```python
from build123d import *

# Parameters (mm, degrees)
BOSS_EXTRUDE2_DEPTH = 2.8956


with BuildPart() as part:
    # Sketch1 → Boss-Extrude2 (new body)
    with BuildSketch(Plane(origin=(0, 0, 0), x_dir=(1, 0, 0), z_dir=(0, 1, 0))):
        with BuildLine():
            Line((21.59, 1.2446), (25.393976036, 1.2446))
            add(Edge.make_bspline(
                [(25.393976036, 1.2446), (25.305125525, 10.422131382), (23.943355437, 19.0754)],
                knots=[4.73416848, 4.73416848, 4.73416848, 5.052697334, 5.052697334, 5.052697334], degree=2, weights=[1, 0.987344206, 1]))
            Line((23.943355437, 19.0754), (19.930240776, 19.0754))
            Line((19.930240776, 19.0754), (19.930240776, 21.5646))
            Line((19.930240776, 21.5646), (23.522368768, 21.5646))
            add(Edge.make_bspline(
                [(23.522368768, 21.5646), (17.413838434, 55.296547713), (1.2446, 57.081350193)],
                knots=[5.099304053, 5.099304053, 5.099304053, 6.234165678, 6.234165678, 6.234165678], degree=2, weights=[1, 0.843284611, 1]))
            Line((1.2446, 57.081350193), (1.2446, 53.34))
            Line((1.2446, 53.34), (-1.2446, 53.34))
            Line((-1.2446, 53.34), (-1.2446, 57.081350193))
            add(Edge.make_bspline(
                [(-1.2446, 57.081350193), (-17.413838434, 55.296547713), (-23.522368768, 21.5646)],
                knots=[0.049019629, 0.049019629, 0.049019629, 1.183881254, 1.183881254, 1.183881254], degree=2, weights=[1, 0.843284611, 1]))
            Line((-23.522368768, 21.5646), (-19.930240776, 21.5646))
            Line((-19.930240776, 21.5646), (-19.930240776, 19.0754))
            Line((-19.930240776, 19.0754), (-23.943355437, 19.0754))
            add(Edge.make_bspline(
                [(-23.943355437, 19.0754), (-25.305125525, 10.422131382), (-25.393976036, 1.2446)],
                knots=[1.230487974, 1.230487974, 1.230487974, 1.549016827, 1.549016827, 1.549016827], degree=2, weights=[1, 0.987344206, 1]))
            Line((-25.393976036, 1.2446), (-21.59, 1.2446))
            Line((-21.59, 1.2446), (-21.59, -1.2446))
            Line((-21.59, -1.2446), (-25.393976036, -1.2446))
            add(Edge.make_bspline(
                [(-25.393976036, -1.2446), (-25.305125525, -10.422131382), (-23.943355437, -19.0754)],
                knots=[1.592575826, 1.592575826, 1.592575826, 1.91110468, 1.91110468, 1.91110468], degree=2, weights=[1, 0.987344206, 1]))
            Line((-23.943355437, -19.0754), (-19.930240776, -19.0754))
            Line((-19.930240776, -19.0754), (-19.930240776, -21.5646))
            Line((-19.930240776, -21.5646), (-23.522368768, -21.5646))
            add(Edge.make_bspline(
                [(-23.522368768, -21.5646), (-22.395811131, -27.785569894), (-20.658836503, -33.249220312)],
                knots=[1.957711399, 1.957711399, 1.957711399, 2.191722412, 2.191722412, 2.191722412], degree=2, weights=[1, 0.993162662, 1]))
            Line((-20.658836503, -33.249220312), (-40.656934115, -75.189915873))
            ThreePointArc((-40.656934115, -75.189915873), (-40.089838211, -78.146952179), (-37.097948163, -78.484969079))
            Line((-37.097948163, -78.484969079), (-8.029094451, -54.219568092))
            add(Edge.make_bspline(
                [(-8.029094451, -54.219568092), (0, -60.238814416), (8.029094451, -54.219568092)],
                knots=[2.819970364, 2.819970364, 2.819970364, 3.463214943, 3.463214943, 3.463214943], degree=2, weights=[1, 0.948723851, 1]))
            Line((8.029094451, -54.219568092), (37.097948163, -78.484969079))
            ThreePointArc((37.097948163, -78.484969079), (40.089838211, -78.146952179), (40.656934115, -75.189915873))
            Line((40.656934115, -75.189915873), (20.658836503, -33.249220312))
            add(Edge.make_bspline(
                [(20.658836503, -33.249220312), (22.395811131, -27.785569894), (23.522368768, -21.5646)],
                knots=[4.091462895, 4.091462895, 4.091462895, 4.325473908, 4.325473908, 4.325473908], degree=2, weights=[1, 0.993162662, 1]))
            Line((23.522368768, -21.5646), (19.930240776, -21.5646))
            Line((19.930240776, -21.5646), (19.930240776, -19.0754))
            Line((19.930240776, -19.0754), (23.943355437, -19.0754))
            add(Edge.make_bspline(
                [(23.943355437, -19.0754), (25.305125525, -10.422131382), (25.393976036, -1.2446)],
                knots=[4.372080627, 4.372080627, 4.372080627, 4.690609481, 4.690609481, 4.690609481], degree=2, weights=[1, 0.987344206, 1]))
            Line((25.393976036, -1.2446), (21.59, -1.2446))
            Line((21.59, -1.2446), (21.59, 1.2446))
        make_face()
        with BuildLine():
            Line((-14.613224312, -41.884600001), (-10.124198394, -41.884600001))
            add(Edge.make_bspline(
                [(0, -50.8), (-0.374242122, -50.8), (-1.087449753, -50.722280744), (-2.740425126, -50.190283538), (-5.318112389, -48.514264833), (-8.117471478, -45.20633596), (-9.696301311, -42.637606864), (-10.124198394, -41.884600001)],
                knots=[-3.141592654, -3.141592654, -3.141592654, -3.141592654, -3.043417883, -2.945243113, -2.748893572, -2.552544031, -2.478028469, -2.478028469, -2.478028469, -2.478028469], degree=3))
            add(Edge.make_bspline(
                [(0, -50.8), (0.374242122, -50.8), (1.087449753, -50.722280744), (2.740425126, -50.190283538), (5.318112389, -48.514264833), (8.117471478, -45.20633596), (9.696301311, -42.637606864), (10.124198394, -41.884600001)],
                knots=[-3.141592654, -3.141592654, -3.141592654, -3.141592654, -3.043417883, -2.945243113, -2.748893572, -2.552544031, -2.478028469, -2.478028469, -2.478028469, -2.478028469], degree=3))
            Line((10.124198394, -41.884600001), (14.613224312, -41.884600001))
            Line((14.613224312, -41.884600001), (14.613224312, -39.395400001))
            Line((14.613224312, -39.395400001), (11.431305901, -39.395400001))
            add(Edge.make_bspline(
                [(11.431305901, -39.395400001), (11.677149239, -38.889598832), (12.987812642, -36.070874709), (15.148196965, -30.166196648), (18.099752632, -17.775460251), (19.683498245, 0), (18.099752632, 17.775460251), (15.148196965, 30.166196648), (12.987812642, 36.070874709), (11.677149239, 38.889598832), (11.431305901, 39.395400001)],
                knots=[-2.400745736, -2.400745736, -2.400745736, -2.400745736, -2.35619449, -2.159844949, -1.963495408, -1.570796327, -1.178097245, -0.981747704, -0.785398163, -0.740846918, -0.740846918, -0.740846918, -0.740846918], degree=3))
            Line((11.431305901, 39.395400001), (14.613224312, 39.395400001))
            Line((14.613224312, 39.395400001), (14.613224312, 41.884600001))
            Line((14.613224312, 41.884600001), (10.124198394, 41.884600001))
            add(Edge.make_bspline(
                [(10.124198394, 41.884600001), (9.696301311, 42.637606864), (8.117471478, 45.20633596), (5.318112389, 48.514264833), (2.740425126, 50.190283538), (1.087449753, 50.722280744), (0.374242122, 50.8), (0, 50.8)],
                knots=[-0.663564185, -0.663564185, -0.663564185, -0.663564185, -0.589048623, -0.392699082, -0.196349541, -0.09817477, 0, 0, 0, 0], degree=3))
            add(Edge.make_bspline(
                [(-10.124198394, 41.884600001), (-9.696301311, 42.637606864), (-8.117471478, 45.20633596), (-5.318112389, 48.514264833), (-2.740425126, 50.190283538), (-1.087449753, 50.722280744), (-0.374242122, 50.8), (0, 50.8)],
                knots=[-0.663564185, -0.663564185, -0.663564185, -0.663564185, -0.589048623, -0.392699082, -0.196349541, -0.09817477, 0, 0, 0, 0], degree=3))
            Line((-10.124198394, 41.884600001), (-14.613224312, 41.884600001))
            Line((-14.613224312, 41.884600001), (-14.613224312, 39.395400001))
            Line((-14.613224312, 39.395400001), (-11.431305901, 39.395400001))
            add(Edge.make_bspline(
                [(-11.431305901, -39.395400001), (-11.677149239, -38.889598832), (-12.987812642, -36.070874709), (-15.148196965, -30.166196648), (-18.099752632, -17.775460251), (-19.683498245, 0), (-18.099752632, 17.775460251), (-15.148196965, 30.166196648), (-12.987812642, 36.070874709), (-11.677149239, 38.889598832), (-11.431305901, 39.395400001)],
                knots=[-2.400745736, -2.400745736, -2.400745736, -2.400745736, -2.35619449, -2.159844949, -1.963495408, -1.570796327, -1.178097245, -0.981747704, -0.785398163, -0.740846918, -0.740846918, -0.740846918, -0.740846918], degree=3))
            Line((-11.431305901, -39.395400001), (-14.613224312, -39.395400001))
            Line((-14.613224312, -39.395400001), (-14.613224312, -41.884600001))
        make_face(mode=Mode.SUBTRACT)
    extrude(amount=BOSS_EXTRUDE2_DEPTH)


solid = part.part
```
Work out the finished part from the listing and answer in its coordinate system (mm). A direction names the side the tool comes from. Round coordinates to 2 decimals unless told otherwise and drop trailing zeros. Write each loop counter-clockwise with the first axis right and the second up, starting at its lowest first coordinate (ties: lowest second). Pieces come first, ordered by that corner, then holes. Notation, with made-up numbers: (-13.75, 62) - (-5.75, 62) arc R12 cw to (-5.75, 82) - close; hole circle Ø8 at (31, 45). An arc over 180 degrees is marked (long way). Return JSON: item names as keys, results as strings. Group by question number.
Q1. The part is cut by section B-B on x = 13. Count the separate pieces of the cut face and the enclosed holes in it, then the cut area to 3 significant figures.
Q2. Each of these flat-tipped pins is pushed along its axis until it touches: pin 1 Ø0.9 at (x, y) = (11.5, 1.5) entering from +Z; pin 2 Ø1.4 at (x, y) = (21.5, 2) entering from +Z; pin 3 Ø1.2 at (x, y) = (-0.5, 1) entering from -Z. Where does it stop, or does it pass through?
Q3. The mould has two halves that part along X. Classify faces 1 (the flat face through (-12, 1, 41.885)), 2 (the flat face through (22, 1, 21.565)), 3 (the flat face through (19.93, 1, 20)): released by +X, released by -X, zero draft, split by the parting line, or undercut.
Q4. The part is cut by section C-C on x = -33. Write down the section's boundary in (y, z).
Q5. For faces 4 (the flat face through (-19.93, 1, -20)), 5 (the flat face through (1.245, 1, -55)), 6 (the flat face through (12, 1, -41.885)), determine the directions among +Z, -Z, +X, -X, +Y, -Y from which every point of the face is accessible in a straight line to the end or side of a thin tool.
Q6. The part is cut by section A-A on x = 31.5. Write down the section's boundary in (y, z).
Q7. Find the intervals of material crossed by L1, parallel to Z at x = 0.5, y = 1.3; L2, parallel to X at y = 0.6, z = 13; L3, parallel to X at y = 1.25, z = 29, in increasing order.
Solved:
{
 "1": {"separate pieces": "4", "enclosed holes": "0", "area": "89.3 mm²"},
 "2": {"pin 1": "z = 57.49", "pin 2": "z = 66.05", "pin 3": "z = -53.34"},
 "3": {"face 1": "undercut", "face 2": "zero draft", "face 3": "released by +X"},
 "4": {"outline": "(0, 59.13) - (2.9, 59.13) - (2.9, 75.06) - (0, 75.06) - close"},
 "5": {"face 4": "-X, +Y, -Y", "face 5": "-Z, +Y, -Y", "face 6": "+Y, -Y"},
 "6": {"outline": "(0, 55.99) - (2.9, 55.99) - (2.9, 73.81) - (0, 73.81) - close"},
 "7": {"L1": "-53.34 to -50.78, 50.78 to 57.14", "L2": "-24.73 to -18.35, 18.35 to 24.73", "L3": "-21.89 to -15.31, 15.31 to 21.89"}
}
